Input: part model. Units: mm. Frame: model coordinates. Give positions to 0.01 mm unless a question says otherwise; leave off trailing zeros. Order: outer loops, then holes, each group sorted by start corner. A loop starts at its lowest first (then second) coordinate and runs counter-clockwise, first axis right, second up. Notation, with made-up numbers: (-36.75, -16) - (21.25, -16) arc R30 ccw to (21.25, 7) - close; hole circle Ø4 at (-5.75, 56.5). An arc over 180 degrees is marked (long way). Answer in a Markdown table with one row per item. Add a question column.
1. Mould query, pull axis X, two halves, no side actions, for faces 1 (the face through (-21.92, -0.99, 2.74)), 2 (the face through (-1.08, -0.99, -4.88)), 3 (the face through (10, -1, 19)). Classes: released by +X, released by -X, zero draft, split by the parting line, or undercut.
2. Contact query for flat-ended pins moving along their axis: pin 1 (0.6 mm diameter, centred on y = -1, z = -16.5, fed in from -X); pin 2 (0.6 mm diameter, centred on x = -22, y = -1.5, fed in from +Z); pin 3 (1 mm diameter, centred on x = -16.5, y = -1.5, fed in from -Z). Output: stop coordinate, or through.
3. Section query B-B on z = 0. Return loops of the section in (x, y), and give its area (3 significant figures).
4. Section query A-A on y = -0.55. Return loops of the section in (x, z).
5. Section query D-D on x = -8. Return loops of the section in (y, z).
6. Ray query, line 1 (Z direction, x = 0, y = -0.5); line 2 (Z direction, x = 0, y = -1.15); line 3 (Z direction, x = 28.5, y = -1.4). Return the intervals inside material, ascending. Write a range as [from, to].
7. Section query C-C on x = 0. Return loops of the section in (y, z).
```python
from build123d import *

# Parameters (mm, degrees)
F0_R         = 5
F1_DEPTH     = 2
F2_T4_DEPTH  = 61.7723426343
F2_T9_DEPTH  = 61.7723426343
F2_T14_DEPTH = 61.7723426343
F2_T19_DEPTH = 61.7723426343


# Not quite as in the source:
# - a fillet or chamfer that OpenCascade refuses, or shapes differently, is made with other operations: its cross-section is extruded or revolved along the edge and cut away or added


with BuildPart() as f1:
    # F0 (on Front) → F1 (new body)
    with BuildSketch(Plane.XZ):
        Polygon((10, 40), (-10, 10), (-40, 10), (-10, -10), (-10, -40), (10, -10), (40, -10), (10, 10), align=None)
        Circle(F0_R, mode=Mode.SUBTRACT)
    extrude(amount=F1_DEPTH)

    # F2: chamfer of 5 on 4 edges, made by hand


with BuildPart() as f2_tool2:
    # F2_s3 → F2_t4 (new body)
    with BuildSketch(Plane(origin=(43.0065402431, 0, -28.6710268287), x_dir=(0, 1, 0), z_dir=(-0.8320502943, 0, 0.5547001962))):
        Polygon((3, -13.8675049056), (-2, -8.8675049056), (-2, -13.8675049056), align=None)
    extrude(amount=F2_T4_DEPTH)

    split(bisect_by=Plane.YZ.offset(10), keep=Keep.TOP)


with BuildPart() as f1_1:
    add(f1.part)

    # F2_t1: cut F2_tool2
    add(f2_tool2.part, mode=Mode.SUBTRACT)


with BuildPart() as f2_tool7:
    # F2_s8 → F2_t9 (new body)
    with BuildSketch(Plane(origin=(28.6710268287, 0, 43.0065402431), x_dir=(0, 1, 0), z_dir=(-0.5547001962, 0, -0.8320502943))):
        Polygon((3, -13.8675049056), (-2, -8.8675049056), (-2, -13.8675049056), align=None)
    extrude(amount=F2_T9_DEPTH)

    split(bisect_by=Plane.XY.offset(10), keep=Keep.TOP)


with BuildPart() as f1_2:
    add(f1_1.part)

    # F2_t6: cut F2_tool7
    add(f2_tool7.part, mode=Mode.SUBTRACT)


with BuildPart() as f2_tool12:
    # F2_s13 → F2_t14 (new body)
    with BuildSketch(Plane(origin=(-43.0065402431, 0, 28.6710268287), x_dir=(0, 1, 0), z_dir=(0.8320502943, 0, -0.5547001962))):
        Polygon((3, -13.8675049056), (-2, -8.8675049056), (-2, -13.8675049056), align=None)
    extrude(amount=F2_T14_DEPTH)

    split(bisect_by=Plane.YZ.offset(-10), keep=Keep.BOTTOM)


with BuildPart() as f1_3:
    add(f1_2.part)

    # F2_t11: cut F2_tool12
    add(f2_tool12.part, mode=Mode.SUBTRACT)


with BuildPart() as f2_tool17:
    # F2_s18 → F2_t19 (new body)
    with BuildSketch(Plane(origin=(-28.6710268287, 0, -43.0065402431), x_dir=(0, 1, 0), z_dir=(0.5547001962, 0, 0.8320502943))):
        Polygon((3, -13.8675049056), (-2, -8.8675049056), (-2, -13.8675049056), align=None)
    extrude(amount=F2_T19_DEPTH)

    split(bisect_by=Plane.XY.offset(-10), keep=Keep.BOTTOM)


with BuildPart() as f1_4:
    add(f1_3.part)

    # F2_t16: cut F2_tool17
    add(f2_tool17.part, mode=Mode.SUBTRACT)


solid = f1_4.part
```
Answer:
| question | item | result |
|---|---|---|
| 1 | face 1 | released by -X |
| 1 | face 2 | undercut |
| 1 | face 3 | released by +X |
| 2 | pin 1 | stops at x = -10 |
| 2 | pin 2 | stops at z = 10 |
| 2 | pin 3 | stops at z = -0.95 |
| 3 | outline | (-19.59, 0) - (-15.99, -2) - (-5, -2) - (-5, 0) - close; (5, -2) - (15.99, -2) - (19.59, 0) - (5, 0) - close |
| 3 | area | 51.2 mm² |
| 4 | outline | (-33.6, 10) - (-10, -5.73) - (-10, -33.6) - (5.73, -10) - (33.6, -10) - (10, 5.73) - (10, 33.6) - (-5.73, 10) - close; hole circle Ø10 at (0, 0) |
| 5 | outline | (-2, -27.99) - (0, -31.59) - (0, 10) - (-2, 10) - close |
| 6 | line 1 | z = [-18.69, -5], [5, 18.69] |
| 6 | line 2 | z = [-17.52, -5], [5, 17.52] |
| 6 | line 3 | z = [-10, -7.62] |
| 7 | outline | (-2, -15.99) - (0, -19.59) - (0, -5) - (-2, -5) - close; (-2, 5) - (0, 5) - (0, 19.59) - (-2, 15.99) - close |
